For this review, take the finished solid that the model builds, in its own axes (mm). Face numbers are marked on the shaded views. A direction names the side the tool comes from. Give positions to 0.01 mm unless a question says otherwise; leave off trailing zeros. Order: outer loops, then holes, each group sorted by start corner. A loop starts at its lowest first (then second) coordinate and runs counter-clockwise, first axis right, second up.
Item 1: For P1, Ø2, axis at x = 5.5, z = 51, coming from the -Y side; P2, Ø24, axis at x = 81.5, y = 8.5, coming from the -Z side; P3, Ø8.5, axis at y = -19.5, z = 20, coming from the -X side, all flat-tipped, find the tip position at first contact; note any pin that passes through.
Item 2: For probe 1 along Y at (x, z) = (-9.5, 40.5); probe 2 along X at (y, z) = (-34, 6.5) (3 decimals); probe 3 along Z at (x, y) = (40.5, 26) (3 decimals), list the stretches that pass through material, from the lowest coordinate up.
Item 3: Consider section C-C (x = 76). Give the boundary of the cut face in (y, z).
Item 4: Machinability: for the marked faces 4, 5, 6, 7 and 8, which of the approach directions +Z, -Z, +X, -X, +Y, -Y give a long, thin tool a straight path to every point of the face, cutting with its end or side? Answer none if there is none.
Item 5: Consider section B-B (y = 44.5). Give the boundary of the cut face in (x, z) (3 decimals).
Item 6: Consider section A-A (z = -2). Give the boundary of the cut face in (x, y) (3 decimals), plus the area to 3 significant figures.
Item 7: The part is to be moulded in two halves that separate along X. For the marked faces 1, 2 and 3, say which applies: released by +X, released by -X, zero draft, split by the parting line, or undercut.
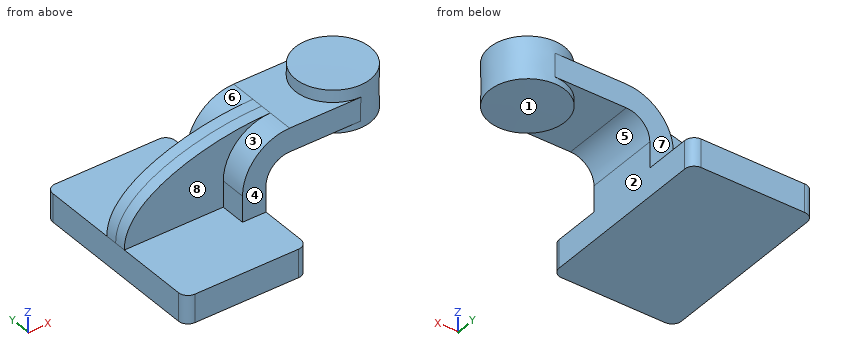
```python
from build123d import *

# Parameters (mm, degrees)
F1_DEPTH = 63.5
F2_DEPTH = 25.4
F3_DEPTH = 7.9375
F4_DEPTH = 25.4
F6_R     = 6.35


with BuildPart() as f1:
    # F0 (on Front) → F1 (new body, symmetric)
    with BuildSketch(Plane.XZ):
        Polygon((-41.275, -9.525), (41.275, -9.525), (41.275, 9.525), (25.4, 9.525), (-41.275, 9.525), align=None)
    extrude(amount=F1_DEPTH, both=True)

    # F0 (on Front) → F2 (join, symmetric)
    with BuildSketch(Plane.XZ):
        with BuildLine():
            Line((25.4, 9.525), (41.275, 9.525))
            Line((41.275, 9.525), (41.275, 27.0002))
            ThreePointArc((41.275, 27.0002), (45.9246798487, 38.2255201513), (57.15, 42.8752))
            Line((57.15, 42.8752), (79.6478510928, 42.8752))
            Line((79.6478510928, 42.8752), (79.6478510928, 58.7502))
            Line((79.6478510928, 58.7502), (57.15, 58.7502))
            ThreePointArc((57.15, 58.7502), (34.6993596973, 49.4508403027), (25.4, 27.0002))
            Line((25.4, 27.0002), (25.4, 9.525))
        make_face()
    extrude(amount=F2_DEPTH, both=True)

    # F0 (on Front) → F3 (join, symmetric)
    with BuildSketch(Plane.XZ):
        with BuildLine():
            add(Edge.make_bspline(
                [(-41.275, 9.525), (-42.0931726694, 43.363686651), (18.200173974, 58.8082894683), (57.15, 58.7502)],
                knots=[0, 0, 0, 0, 110.0481755416, 110.0481755416, 110.0481755416, 110.0481755416], degree=3))
            Line((-41.275, 9.525), (25.4, 9.525))
            Line((25.4, 9.525), (25.4, 27.0002))
            ThreePointArc((25.4, 27.0002), (34.6993596973, 49.4508403027), (57.15, 58.7502))
        make_face()
    extrude(amount=F3_DEPTH, both=True)

    # F0 (on Front) → F4 (join, symmetric)
    with BuildSketch(Plane.XZ):
        Polygon((105.17556149, 58.7502), (79.6478510928, 58.7502), (79.6478510928, 42.8752), (105.0773831404, 42.8752), align=None)
    extrude(amount=F4_DEPTH, both=True)

    # F0 (on Front) → F5 (revolve)
    with BuildSketch(Plane.XZ):
        Polygon((105.2245721221, 66.675), (105.17556149, 58.7502), (105.0773831404, 42.8752), (105.0478510928, 38.1), (130.4478510928, 38.1), (130.4478510928, 66.675), align=None)
    revolve(axis=Axis((105.1362116075, 0, 52.3875), (0.0061843447, 0, 0.9999808768)))

    # F6
    f6_edges = [f1.edges().sort_by_distance(p)[0] for p in [
        (-41.275, -63.5, 0),
        (41.275, -63.5, 0),
        (41.275, 63.5, 0),
        (-41.275, 63.5, 0),
    ]]
    fillet(f6_edges, radius=F6_R)


solid = f1.part
```
Resolved:
1. P1: stops at y = -7.94
1. P2: stops at z = 38.25
1. P3: stops at x = 25.4
2. probe 1: y = -7.94 to 7.94
2. probe 2: x = -41.275 to 41.275
2. probe 3: z = -9.525 to 9.525
3. outline: (-25.4, 42.88) - (25.4, 42.88) - (25.4, 58.75) - (-25.4, 58.75) - close
4. face 4: +Z, +X, -X, -Y
4. face 5: -Z, +Y, -Y
4. face 6: +Z, -X, +Y
4. face 7: +Z, +X, -X, +Y
4. face 8: +Z, -X, -Y
5. outline: (-41.275, -9.525) - (41.275, -9.525) - (41.275, 9.525) - (-41.275, 9.525) - close
6. outline: (-41.275, -57.15) arc R6.35 ccw to (-34.925, -63.5) - (34.925, -63.5) arc R6.35 ccw to (41.275, -57.15) - (41.275, 57.15) arc R6.35 ccw to (34.925, 63.5) - (-34.925, 63.5) arc R6.35 ccw to (-41.275, 57.15) - close
6. area: 10,400 mm2
7. face 1: undercut
7. face 2: released by +X
7. face 3: released by -X
